from build123d import *

# Parameters (mm, degrees)
F1_DEPTH = 64
F3_DEPTH = 25
F4_T     = -3
F5_R     = 9.5
F6_DEPTH = 3


with BuildPart() as f1:
    # F0 (on Front) → F1 (new body)
    with BuildSketch(Plane.XZ):
        Polygon((-45, 77.9422863406), (0, 0), (140, 0), (140, 19), (10.9696551146, 19), (-19.0455173281, 70.9878036687), (36.3801085141, 102.9878036687), (26.8801085141, 119.4422863406), align=None)
    extrude(amount=-F1_DEPTH)

    # F2 (on face) → F3 (cut)
    with BuildSketch(Plane(origin=(-45, 0, 77.9422863406), x_dir=(0.8660254038, 0, 0.5), z_dir=(-0.5, 0, 0.8660254038))):
        with BuildLine():
            ThreePointArc((51, 64), (73.627416998, 54.627416998), (83, 32))
            Line((83, 32), (83, 64))
            Line((83, 64), (51, 64))
        make_face()
        with BuildLine():
            Line((83, 0), (83, 32))
            ThreePointArc((83, 32), (73.627416998, 9.372583002), (51, 0))
            Line((51, 0), (83, 0))
        make_face()
    extrude(amount=-F3_DEPTH, mode=Mode.SUBTRACT)

    # F4
    f4_openings = [f1.faces().sort_by_distance(p)[0] for p in [
        (-11.74342, 32, 97.142982),
    ]]
    offset(amount=F4_T, openings=f4_openings, kind=Kind.INTERSECTION)

    # F5 (on face) → F6 (cut, through all)
    with BuildSketch(Plane(origin=(-37, 0, 64.08587988), x_dir=(0.8660254038, 0, 0.5), z_dir=(-0.5, 0, 0.8660254038))):
        with Locations((51, 32)):
            Circle(F5_R)
    extrude(amount=-F6_DEPTH, mode=Mode.SUBTRACT)


solid = f1.part
CAD build for the part. Positions are in the model's coordinates, mm. A direction names the side the tool comes from. Round coordinates to 2 decimals unless told otherwise and drop trailing zeros. Loops run counter-clockwise (first coordinate to the right, second up) from the corner with the lowest first, then second, coordinate; pieces in that order, holes last.
(1) Cut at A-A (x = 90). Give the cut face in (y, z).
(2) Cut at B-B (y = 27). Give the cut face in (x, z), plus the area to 3 significant figures.
(3) Wall check: line 1 along Z through (x, y) = (57, 12.5); line 2 along Z through (x, y) = (20, 16); line 3 along Y through (x, z) = (-17, 77). Give the ranges that are in metal, low to high.
(4) Which spindle directions (+Z, -Z, +X, -X, +Y, -Y) get a long thin tool onto all of the face, cutting with end or side? Do faces 5 (the flat face through (76, 32, 19)), 6 (the flat face through (-14.217, 62.665, 95.715)), 7 (the flat face through (27, 61, 13)). Say none if no direction does.
(5) Two-plate mould, pull along X, no slides. Class faces 1 (the flat face through (-6.726, 31.594, 43.65)), 2 (the flat face through (27, 64, 17)), 3 (the flat face through (-22.815, 31.552, 39.517)), 4 (the flat face through (137, 32, 9)): +X half, -X half, draft (parallel to the pull), parting line (faces both ways), or undercut.
(6) Drop flat-ended pins along their axis: pin 1 (8 mm diameter, centred on y = 29.5, z = 57, fed in from +X); pin 2 (3 mm diameter, centred on y = 19, z = 20, fed in from +X); pin 3 (10.5 mm diameter, centred on y = 37, z = 7, fed in from -X); pin 4 (2 mm diameter, centred on y = 9, z = 102, fed in from +X). Give the stop position or say it passes through.
(7) Cut at D-D (y = 13). Give the cut face in (x, z), plus the area to 3 significant figures.
(8) Cut at C-C (z = 10). Give the cut face in (x, y), plus the area to 3 significant figures.
Findings below:
1. outline: (0, 0) - (64, 0) - (64, 19) - (0, 19) - close; hole (3, 3) - (61, 3) - (61, 16) - (3, 16) - close
2. outline: (-45, 77.94) - (0, 0) - (140, 0) - (140, 19) - (10.97, 19) - (-19.05, 70.99) - (1.67, 82.95) - (0.17, 85.55) - (-23.14, 72.09) - (9.24, 16) - (137, 16) - (137, 3) - (1.73, 3) - (-42.4, 79.44) - close; (14.16, 93.62) - (15.66, 91.03) - (36.04, 102.79) - (26.54, 119.25) - (23.91, 117.73) - (31.91, 103.87) - close
2. area: 1,500 mm2
3. line 1: z = 0 to 3, 16 to 19
3. line 2: z = 0 to 3, 16 to 19, 93.53 to 96.99
3. line 3: y = 0 to 3, 61 to 64
4. face 5: +X, +Y, -Y
4. face 6: +Z, -X, +Y, -Y
4. face 7: none
5. face 1: undercut
5. face 2: draft
5. face 3: -X half
5. face 4: undercut
6. pin 1: stops at x = -8.66
6. pin 2: stops at x = 140
6. pin 3: stops at x = -7.07
6. pin 4: stops at x = 26.98
7. outline: (-45, 77.94) - (0, 0) - (140, 0) - (140, 19) - (10.97, 19) - (-19.05, 70.99) - (30.97, 99.86) - (21.47, 116.32) - (18.14, 114.4) - (26.14, 100.54) - (-23.14, 72.09) - (9.24, 16) - (137, 16) - (137, 3) - (1.73, 3) - (-42.4, 79.44) - close
7. area: 1,540 mm2
8. outline: (-5.77, 0) - (140, 0) - (140, 64) - (-5.77, 64) - close; hole (-2.31, 3) - (137, 3) - (137, 61) - (-2.31, 61) - close
8. area: 1,250 mm2
